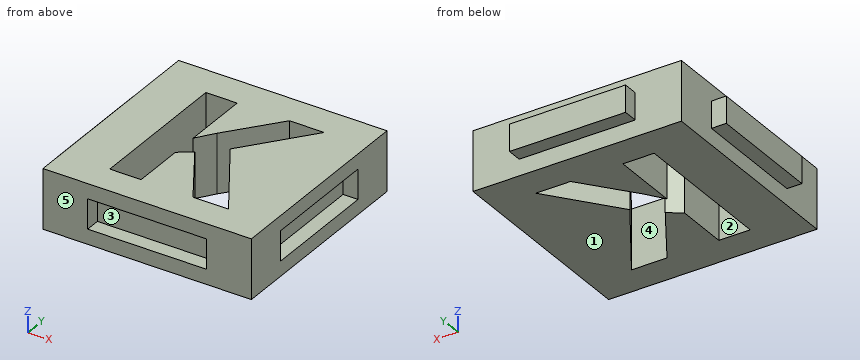
from build123d import *

# Parameters (mm, degrees)
F0_W     = 35.56
F0_H     = 35.56
F1_DEPTH = 5.08
F2_W     = 19.812
F2_H     = 4.572
F3_DEPTH = 2.54
F4_W     = 19.812
F4_H     = 4.572
F5_DEPTH = 2.54
F6_W     = 20.32
F6_H     = 5.08
F7_DEPTH = 2.54
F8_W     = 20.32
F8_H     = 5.08
F9_DEPTH = 2.54


with BuildPart() as f1:
    # F0 (on Top) → F1 (new body, symmetric)
    with BuildSketch(Plane.XY):
        Rectangle(F0_W, F0_H)
        Polygon((1.7170355903, 1.339453125), (10.5695529514, -12.7), (4.5061848958, -12.7), (-2.0918619792, -2.0891059028), (-4.3463324653, -3.7096788194), (-4.3463324653, -12.7), (-9.6876085069, -12.7), (-9.6876085069, 12.4850260417), (-4.3463324653, 12.4850260417), (-4.3463324653, 0.9591145833), (-2.2462022569, 3.9246527778), (4.5778428819, 12.4850260417), (10.5034071181, 12.4850260417), align=None, mode=Mode.SUBTRACT)
    extrude(amount=F1_DEPTH, both=True)

    # F2 (on face) → F3 (join)
    with BuildSketch(Plane(origin=(0, 17.78, 0), x_dir=(-1, 0, 0), z_dir=(0, 1, 0))):
        Rectangle(F2_W, F2_H)
    extrude(amount=F3_DEPTH)

    # F4 (on face) → F5 (join)
    with BuildSketch(Plane(origin=(-17.78, 0, 0), x_dir=(0, -1, 0), z_dir=(-1, 0, 0))):
        Rectangle(F4_W, F4_H)
    extrude(amount=F5_DEPTH)

    # F6 (on face) → F7 (cut)
    with BuildSketch(Plane.XZ.offset(17.78)):
        Rectangle(F6_W, F6_H)
    extrude(amount=-F7_DEPTH, mode=Mode.SUBTRACT)

    # F8 (on face) → F9 (cut)
    with BuildSketch(Plane.YZ.offset(17.78)):
        Rectangle(F8_W, F8_H)
    extrude(amount=-F9_DEPTH, mode=Mode.SUBTRACT)


solid = f1.part
For this review, take the finished solid that the model builds, in its own axes (mm). Face numbers are marked on the shaded views. A direction names the side the tool comes from. Round coordinates to 2 decimals unless told otherwise and drop trailing zeros. Write each loop counter-clockwise with the first axis right and the second up, starting at its lowest first coordinate (ties: lowest second). Pieces come first, ordered by that corner, then holes. Notation, with made-up numbers: M 54.5,15 L 89.5,15 A18 cw 89.5,38 Z; hole C -16.75,33 d2. An arc over 180 degrees is marked long. Write item = value, one per line. Start each with the question number.
(1) We need section C-C (y = 0). Give the boundary of the cut face in (x, z), then the cut area to 3 significant figures.
(2) We need section B-B (x = -6.5). Give the boundary of the cut face in (y, z), then the cut area to 3 significant figures.
(3) We need section D-D (x = 3.5). Give the boundary of the cut face in (y, z), then the cut area to 3 significant figures.
(4) The part is to be moulded in two halves that separate along Z. For the marked faces 1, 2 and 3, say which applies: +Z half, -Z half, draft (parallel to the pull), parting line (faces both ways), or undercut.
(5) For line 1 along Y through (x, z) = (-6, -3.75); line 2 along X through (y, z) = (-8.5, -4); line 3 along X through (y, z) = (5, 0), list the stretches that pass through material, from the lowest coordinate up.
(6) For the marked faces 4 and 5, list the 3-axis set-ups (+Z, -Z, +X, -X, +Y, -Y) from which the entire face can be reached by the end or side of a thin tool; tool diameter is ignored.
(7) Clearance check with flat-ended pins moving along their axes: pin 1 Ø0.8 at (y, z) = (-16.5, 0.5) entering from -X; pin 2 Ø6 at (x, z) = (14, -3) entering from +Y; pin 3 Ø2 at (x, z) = (-19, -0.5) entering from +Y; pin 4 Ø2 at (x, y) = (-2.5, 1.5) entering from +Z. State where each tip first meets the part, or that it passes through.
Results found:
q1.outline = M -20.32,-2.29 L -17.78,-2.29 L -17.78,-5.08 L -9.69,-5.08 L -9.69,5.08 L -17.78,5.08 L -17.78,2.29 L -20.32,2.29 Z; M 2.56,-5.08 L 17.78,-5.08 L 17.78,-2.54 L 15.24,-2.54 L 15.24,2.54 L 17.78,2.54 L 17.78,5.08 L 2.56,5.08 Z
q1.area = 236 mm²
q2.outline = M -17.78,-5.08 L -12.7,-5.08 L -12.7,5.08 L -17.78,5.08 L -17.78,2.54 L -15.24,2.54 L -15.24,-2.54 L -17.78,-2.54 Z; M 12.49,-5.08 L 17.78,-5.08 L 17.78,-2.29 L 20.32,-2.29 L 20.32,2.29 L 17.78,2.29 L 17.78,5.08 L 12.49,5.08 Z
q2.area = 104 mm²
q3.outline = M -17.78,-5.08 L -11.08,-5.08 L -11.08,5.08 L -17.78,5.08 L -17.78,2.54 L -15.24,2.54 L -15.24,-2.54 L -17.78,-2.54 Z; M -1.49,-5.08 L 3.6,-5.08 L 3.6,5.08 L -1.49,5.08 Z; M 11.13,-5.08 L 17.78,-5.08 L 17.78,-2.29 L 20.32,-2.29 L 20.32,2.29 L 17.78,2.29 L 17.78,5.08 L 11.13,5.08 Z
q3.area = 186 mm²
q4.face_1 = -Z half
q4.face_2 = draft
q4.face_3 = undercut
q5.line_1 = -17.78 to -12.7, 12.49 to 17.78
q5.line_2 = -17.78 to -9.69, -4.35 to 1.89, 7.92 to 17.78
q5.line_3 = -20.32 to -9.69, -4.35 to -1.39, 4.6 to 15.24
q6.face_4 = +Z, -Z
q6.face_5 = +Z, -Z, +X, -X, -Y
q7.pin_1 = -17.78
q7.pin_2 = 17.78
q7.pin_3 = 9.91
q7.pin_4 = through
